Verification items for the finished model (mm, model axes). A direction names the side the tool comes from. Coordinates: 2 decimals unless noted, no trailing zeros. Write each loop counter-clockwise with the first axis right and the second up, starting at its lowest first coordinate (ties: lowest second). Pieces come first, ordered by that corner, then holes. Notation, with made-up numbers: (84, 7.25) -> (101, 7.25) arc R28 ccw to (101, 42.25) -> close; hole circle Ø6 at (21, -32.5). An arc over 180 degrees is marked (long way). Answer in a Markdown table with one row per item.
```python
from build123d import *

# Parameters (mm, degrees)
F0_W     = 19.304
F0_H     = 19.4056
F1_DEPTH = 25.4
F2_DEPTH = 15.24
F3_R     = 6.604
F4_DEPTH = 127
F5_R     = 5.08
F6_R     = 5.08


with BuildPart() as f1:
    # F0 (on Front) → F1 (new body)
    with BuildSketch(Plane.XZ):
        with BuildLine():
            Line((-22.225, -9.525), (-22.225, -22.225))
            Line((-22.225, -22.225), (-9.525, -22.225))
            ThreePointArc((-9.525, -22.225), (0, -24.18008), (9.525, -22.225))
            Line((9.525, -22.225), (22.225, -22.225))
            Line((22.225, -22.225), (22.225, -9.525))
            ThreePointArc((22.225, -9.525), (24.18008, 0), (22.225, 9.525))
            Line((22.225, 9.525), (22.225, 22.225))
            Line((22.225, 22.225), (9.525, 22.225))
            ThreePointArc((9.525, 22.225), (0, 24.18008), (-9.525, 22.225))
            Line((-9.525, 22.225), (-22.225, 22.225))
            Line((-22.225, 22.225), (-22.225, 9.525))
            ThreePointArc((-22.225, 9.525), (-24.18008, 0), (-22.225, -9.525))
        make_face()
        Rectangle(F0_W, F0_H, mode=Mode.SUBTRACT)
    extrude(amount=F1_DEPTH)

    # F0 (on Front) → F2 (join)
    with BuildSketch(Plane.XZ):
        Rectangle(F0_W, F0_H)
    extrude(amount=F2_DEPTH)

    # F3 (on face) → F4 (cut)
    with BuildSketch(Plane.XZ.offset(15.24)):
        Circle(F3_R)
    extrude(amount=-F4_DEPTH, mode=Mode.SUBTRACT)

    # F5
    f5_edges = [f1.edges().sort_by_distance(p)[0] for p in [
        (-22.225, -12.7, -22.225),
        (-22.225, -12.7, 22.225),
        (22.225, -12.7, 22.225),
        (22.225, -12.7, -22.225),
    ]]
    fillet(f5_edges, radius=F5_R)

    # F6
    f6_edges = [f1.edges().sort_by_distance(p)[0] for p in [
        (-13.335, -25.4, -22.225),
        (-13.335, 0, -22.225),
        (-13.335, 0, 22.225),
        (-22.225, -25.4, 13.335),
        (22.225, -25.4, 13.335),
        (22.225, -25.4, -13.335),
        (13.335, 0, -22.225),
        (13.335, 0, 22.225),
        (0, -25.4, -24.18008),
        (0, 0, -24.18008),
        (0, 0, 24.18008),
        (0, -25.4, 24.18008),
        (24.18008, -25.4, 0),
        (24.18008, 0, 0),
        (-24.18008, 0, 0),
        (-24.18008, -25.4, 0),
    ]]
    fillet(f6_edges, radius=F6_R)


solid = f1.part
```
1. Access from +Z, -Z, +X, -X, +Y, -Y to the whole of each face (thin tool, end or side, straight path). Record for faces 1 (the face through (-20.7, -1.45, 12.72)), 2 (the face through (-22.225, -13, 13)), 3 (the face through (-22.225, -13, -13)), 4 (the face through (20.78, -23.87, -12.72)), 5 (the face through (20.7, -1.45, -12.72)).
Findings below:
| item | result |
|---|---|
| face 1 | +Z, -X, +Y |
| face 2 | +Z, -X, +Y, -Y |
| face 3 | -Z, -X, +Y, -Y |
| face 4 | -Z, +X, -Y |
| face 5 | -Z, +X, +Y |
2. Sectioned sample at A-A, the plane x = 0. Record the cut outline in (y, z).
Findings below:
| item | result |
|---|---|
| outline | (-25.4, -19.1) arc R5.08 ccw to (-20.32, -24.18) -> (-5.08, -24.18) arc R5.08 ccw to (0, -19.1) -> (0, -6.6) -> (-15.24, -6.6) -> (-15.24, -9.7) -> (-25.4, -9.7) -> close; (-25.4, 9.7) -> (-15.24, 9.7) -> (-15.24, 6.6) -> (0, 6.6) -> (0, 19.1) arc R5.08 ccw to (-5.08, 24.18) -> (-20.32, 24.18) arc R5.08 ccw to (-25.4, 19.1) -> close |
3. Sectioned sample at B-B, the plane y = -10.5. Record the cut outline in (x, z) (3 decimals).
Findings below:
| item | result |
|---|---|
| outline | (-22.225, -17.145) arc R5.08 ccw to (-17.145, -22.225) -> (-9.525, -22.225) arc R24.18 ccw to (9.525, -22.225) -> (17.145, -22.225) arc R5.08 ccw to (22.225, -17.145) -> (22.225, -9.525) arc R24.18 ccw to (22.225, 9.525) -> (22.225, 17.145) arc R5.08 ccw to (17.145, 22.225) -> (9.525, 22.225) arc R24.18 ccw to (-9.525, 22.225) -> (-17.145, 22.225) arc R5.08 ccw to (-22.225, 17.145) -> (-22.225, 9.525) arc R24.18 ccw to (-22.225, -9.525) -> close; hole circle Ø13.208 at (0, 0) |
4. Go/stop test with flat-tipped pins: pin 1 (1.5 mm diameter, centred on y = -19, z = -10, fed in from -X); pin 2 (11 mm diameter, centred on y = -22, z = -2, fed in from -X); pin 3 (4 mm diameter, centred on x = 13, y = -15, fed in from -Z) (3 decimals). Record where each tip stops, or that it passes through.
Findings below:
| item | result |
|---|---|
| pin 1 | stops at x = -22.34 |
| pin 2 | stops at x = -24.18 |
| pin 3 | stops at z = -22.225 |
5. Sectioned sample at D-D, the plane z = -13.5. Record the cut outline in (x, y) (3 decimals).
Findings below:
| item | result |
|---|---|
| outline | (-22.225, -20.32) arc R5.08 ccw to (-17.145, -25.4) -> (17.145, -25.4) arc R5.08 ccw to (22.225, -20.32) -> (22.225, -5.08) arc R5.08 ccw to (17.145, 0) -> (-17.145, 0) arc R5.08 ccw to (-22.225, -5.08) -> close |
6. Release check for a two-part mould opening along X. For faces 6 (the face through (-20.776, -12.807, -20.697)), 7 (the face through (0, -15.24, 7)), 8 (the face through (-0.14, -12.59, -24.18)) record: released by +X, released by -X, zero draft, split by the parting line, or undercut.
Findings below:
| item | result |
|---|---|
| face 6 | released by -X |
| face 7 | undercut |
| face 8 | split by the parting line |
7. Sectioned sample at C-C, the plane z = 0. Record the cut outline in (x, y).
Findings below:
| item | result |
|---|---|
| outline | (-24.18, -20.32) arc R5.08 ccw to (-19.1, -25.4) -> (-9.65, -25.4) -> (-9.65, -15.24) -> (-6.6, -15.24) -> (-6.6, 0) -> (-19.1, 0) arc R5.08 ccw to (-24.18, -5.08) -> close; (6.6, -15.24) -> (9.65, -15.24) -> (9.65, -25.4) -> (19.1, -25.4) arc R5.08 ccw to (24.18, -20.32) -> (24.18, -5.08) arc R5.08 ccw to (19.1, 0) -> (6.6, 0) -> close |
8. Material ranges on probe 1 along Z at (x, y) = (0, -6.5); probe 2 along Z at (x, y) = (-14, -6.75) (3 decimals); probe 3 along X at (y, z) = (-13.25, -2), recorded low to high. Write a range as from..to.
Findings below:
| item | result |
|---|---|
| probe 1 | z = -24.18..-6.6, 6.6..24.18 |
| probe 2 | z = -22.225..22.225 |
| probe 3 | x = -24.1..-6.29, 6.29..24.1 |
